from build123d import *

# Parameters (mm, degrees)
SKETCH11_R                             = 2.5
F_25_SERIES_EXTRUSIONS_25_2550_1_DEPTH = 170


with BuildPart() as part:
    # Sketch11 → 25 series extrusions 25-2550(1) (new body)
    with BuildSketch(Plane(origin=(0, 0, 0), x_dir=(-1, 0, 0), z_dir=(0, 1, 0))):
        with BuildLine():
            Line((8.185, 12.5), (-8.185, 12.5))
            ThreePointArc((-8.185, 12.5), (-9.25, 11.435), (-8.185, 10.37))
            Line((-8.185, 10.37), (-6.227198013, 10.37))
            ThreePointArc((-6.227198013, 10.37), (-5.236616214, 9.708114403), (-5.469039527, 8.539643501))
            Line((-5.469039527, 8.539643501), (-8.697639148, 5.311043881))
            ThreePointArc((-8.697639148, 5.311043881), (-9.72768328, 4.622790395), (-10.942703178, 4.381107911))
            Line((-10.942703178, 4.381107911), (-14.057296822, 4.381107911))
            ThreePointArc((-14.057296822, 4.381107911), (-15.27231672, 4.622790395), (-16.302360852, 5.311043881))
            Line((-16.302360852, 5.311043881), (-19.530960473, 8.539643501))
            ThreePointArc((-19.530960473, 8.539643501), (-19.763383786, 9.708114403), (-18.772801987, 10.37))
            Line((-18.772801987, 10.37), (-16.815, 10.37))
            ThreePointArc((-16.815, 10.37), (-15.75, 11.435), (-16.815, 12.5))
            Line((-16.815, 12.5), (-23, 12.5))
            ThreePointArc((-23, 12.5), (-24.414213562, 11.914213562), (-25, 10.5))
            Line((-25, 10.5), (-25, 4.315))
            ThreePointArc((-25, 4.315), (-23.935, 3.25), (-22.87, 4.315))
            Line((-22.87, 4.315), (-22.87, 6.272801987))
            ThreePointArc((-22.87, 6.272801987), (-22.208114403, 7.263383786), (-21.039643501, 7.030960473))
            Line((-21.039643501, 7.030960473), (-17.811043881, 3.802360852))
            ThreePointArc((-17.811043881, 3.802360852), (-17.122790395, 2.77231672), (-16.881107911, 1.557296822))
            Line((-16.881107911, 1.557296822), (-16.881107911, -1.557296822))
            ThreePointArc((-16.881107911, -1.557296822), (-17.122790395, -2.77231672), (-17.811043881, -3.802360852))
            Line((-17.811043881, -3.802360852), (-21.039643501, -7.030960473))
            ThreePointArc((-21.039643501, -7.030960473), (-22.208114403, -7.263383786), (-22.87, -6.272801987))
            Line((-22.87, -6.272801987), (-22.87, -4.315))
            ThreePointArc((-22.87, -4.315), (-23.935, -3.25), (-25, -4.315))
            Line((-25, -4.315), (-25, -10.5))
            ThreePointArc((-25, -10.5), (-24.414213562, -11.914213562), (-23, -12.5))
            Line((-23, -12.5), (-16.815, -12.5))
            ThreePointArc((-16.815, -12.5), (-15.75, -11.435), (-16.815, -10.37))
            Line((-16.815, -10.37), (-18.772801987, -10.37))
            ThreePointArc((-18.772801987, -10.37), (-19.763383786, -9.708114403), (-19.530960473, -8.539643501))
            Line((-19.530960473, -8.539643501), (-16.302360852, -5.311043881))
            ThreePointArc((-16.302360852, -5.311043881), (-15.27231672, -4.622790395), (-14.057296822, -4.381107911))
            Line((-14.057296822, -4.381107911), (-10.942703178, -4.381107911))
            ThreePointArc((-10.942703178, -4.381107911), (-9.72768328, -4.622790395), (-8.697639148, -5.311043881))
            Line((-8.697639148, -5.311043881), (-5.469039527, -8.539643501))
            ThreePointArc((-5.469039527, -8.539643501), (-5.236616214, -9.708114403), (-6.227198013, -10.37))
            Line((-6.227198013, -10.37), (-8.185, -10.37))
            ThreePointArc((-8.185, -10.37), (-9.25, -11.435), (-8.185, -12.5))
            Line((-8.185, -12.5), (8.185, -12.5))
            ThreePointArc((8.185, -12.5), (9.25, -11.435), (8.185, -10.37))
            Line((8.185, -10.37), (6.227198013, -10.37))
            ThreePointArc((6.227198013, -10.37), (5.236616214, -9.708114403), (5.469039527, -8.539643501))
            Line((5.469039527, -8.539643501), (8.697639148, -5.311043881))
            ThreePointArc((8.697639148, -5.311043881), (9.72768328, -4.622790395), (10.942703178, -4.381107911))
            Line((10.942703178, -4.381107911), (14.057296822, -4.381107911))
            ThreePointArc((14.057296822, -4.381107911), (15.27231672, -4.622790395), (16.302360852, -5.311043881))
            Line((16.302360852, -5.311043881), (19.530960473, -8.539643501))
            ThreePointArc((19.530960473, -8.539643501), (19.763383786, -9.708114403), (18.772801987, -10.37))
            Line((18.772801987, -10.37), (16.815, -10.37))
            ThreePointArc((16.815, -10.37), (15.75, -11.435), (16.815, -12.5))
            Line((16.815, -12.5), (23, -12.5))
            ThreePointArc((23, -12.5), (24.414213562, -11.914213562), (25, -10.5))
            Line((25, -10.5), (25, -4.315))
            ThreePointArc((25, -4.315), (23.935, -3.25), (22.87, -4.315))
            Line((22.87, -4.315), (22.87, -6.272801987))
            ThreePointArc((22.87, -6.272801987), (22.208114403, -7.263383786), (21.039643501, -7.030960473))
            Line((21.039643501, -7.030960473), (17.811043881, -3.802360852))
            ThreePointArc((17.811043881, -3.802360852), (17.122790395, -2.77231672), (16.881107911, -1.557296822))
            Line((16.881107911, -1.557296822), (16.881107911, 1.557296822))
            ThreePointArc((16.881107911, 1.557296822), (17.122790395, 2.77231672), (17.811043881, 3.802360852))
            Line((17.811043881, 3.802360852), (21.039643501, 7.030960473))
            ThreePointArc((21.039643501, 7.030960473), (22.208114403, 7.263383786), (22.87, 6.272801987))
            Line((22.87, 6.272801987), (22.87, 4.315))
            ThreePointArc((22.87, 4.315), (23.935, 3.25), (25, 4.315))
            Line((25, 4.315), (25, 10.5))
            ThreePointArc((25, 10.5), (24.414213562, 11.914213562), (23, 12.5))
            Line((23, 12.5), (16.815, 12.5))
            ThreePointArc((16.815, 12.5), (15.75, 11.435), (16.815, 10.37))
            Line((16.815, 10.37), (18.772801987, 10.37))
            ThreePointArc((18.772801987, 10.37), (19.763383786, 9.708114403), (19.530960473, 8.539643501))
            Line((19.530960473, 8.539643501), (16.302360852, 5.311043881))
            ThreePointArc((16.302360852, 5.311043881), (15.27231672, 4.622790395), (14.057296822, 4.381107911))
            Line((14.057296822, 4.381107911), (10.942703178, 4.381107911))
            ThreePointArc((10.942703178, 4.381107911), (9.72768328, 4.622790395), (8.697639148, 5.311043881))
            Line((8.697639148, 5.311043881), (5.469039527, 8.539643501))
            ThreePointArc((5.469039527, 8.539643501), (5.236616214, 9.708114403), (6.227198013, 10.37))
            Line((6.227198013, 10.37), (8.185, 10.37))
            ThreePointArc((8.185, 10.37), (9.25, 11.435), (8.185, 12.5))
        make_face()
        with Locations((-12.5, 0)):
            Circle(SKETCH11_R, mode=Mode.SUBTRACT)
        with Locations((12.5, 0)):
            Circle(SKETCH11_R, mode=Mode.SUBTRACT)
        with BuildLine():
            Line((-1.678781255, 10.37), (1.678781255, 10.37))
            ThreePointArc((1.678781255, 10.37), (2.198638297, 10.16512894), (2.438958165, 9.660678886))
            ThreePointArc((2.438958165, 9.660678886), (2.716823224, 8.564426963), (3.361297928, 7.635110212))
            Line((3.361297928, 7.635110212), (7.191171941, 3.805236199))
            ThreePointArc((7.191171941, 3.805236199), (7.879425427, 2.775192067), (8.121107911, 1.560172169))
            Line((8.121107911, 1.560172169), (8.121107911, -1.560172169))
            ThreePointArc((8.121107911, -1.560172169), (7.879425427, -2.775192067), (7.191171941, -3.805236199))
            Line((7.191171941, -3.805236199), (3.361297928, -7.635110212))
            ThreePointArc((3.361297928, -7.635110212), (2.716823224, -8.564426963), (2.438958165, -9.660678886))
            ThreePointArc((2.438958165, -9.660678886), (2.198638297, -10.16512894), (1.678781255, -10.37))
            Line((1.678781255, -10.37), (-1.678781255, -10.37))
            ThreePointArc((-1.678781255, -10.37), (-2.198638297, -10.16512894), (-2.438958165, -9.660678886))
            ThreePointArc((-2.438958165, -9.660678886), (-2.716823224, -8.564426963), (-3.361297928, -7.635110212))
            Line((-3.361297928, -7.635110212), (-7.191171941, -3.805236199))
            ThreePointArc((-7.191171941, -3.805236199), (-7.879425427, -2.775192067), (-8.121107911, -1.560172169))
            Line((-8.121107911, -1.560172169), (-8.121107911, 1.560172169))
            ThreePointArc((-8.121107911, 1.560172169), (-7.879425427, 2.775192067), (-7.191171941, 3.805236199))
            Line((-7.191171941, 3.805236199), (-3.361297928, 7.635110212))
            ThreePointArc((-3.361297928, 7.635110212), (-2.716823224, 8.564426963), (-2.438958165, 9.660678886))
            ThreePointArc((-2.438958165, 9.660678886), (-2.198638297, 10.16512894), (-1.678781255, 10.37))
        make_face(mode=Mode.SUBTRACT)
    extrude(amount=F_25_SERIES_EXTRUSIONS_25_2550_1_DEPTH)


solid = part.part
Here's how the part is built. I have some questions about the finished solid (model axes, mm). A direction names the side the tool comes from. Give positions to 0.01 mm unless a question says otherwise; leave off trailing zeros. Write each loop counter-clockwise with the first axis right and the second up, starting at its lowest first coordinate (ties: lowest second). Pieces come first, ordered by that corner, then holes. Notation, with made-up numbers: (33, 19) -> (91, 19) arc R9 ccw to (91, 27) -> close; hole circle Ø6 at (67, 41). An arc over 180 degrees is marked (long way). Use one line per item in the form item = value. Start each with the question number.
1. Will these pins go through, and if not, where does the flat tip stop? pin 1 Ø3.5 at (x, y) = (13, 52.5) entering from -Z; pin 2 Ø3.5 at (x, y) = (12, 49) entering from +Z; pin 3 Ø2.5 at (x, y) = (-12.5, 50.5) entering from +Z; pin 4 Ø3 at (x, z) = (-2, -4.5) entering from +Y.
2. Imagine slicing it at B-B on x = 12.5. List the corners of the cut face in (y, z) for me.
3. On a 3-axis mill with a long thin cutter (end or side, diameter ignored), from which of +Z, -Z, +X, -X, +Y, -Y can I reach the whole of each face in a straight line? I mean faces 1 (the face through (-12, 84, -4.381)), 2 (the face through (-7.06, 83.81, -6.95)), 3 (the face through (-16.881, 84, 0)), 4 (the face through (-13, 84, 4.381)). Say none if no direction works.
4. Imagine slicing it at A-A on z = 0. List the corners of the cut face in (x, y) for me, plus the area to 3 significant figures.
5. Thinking about a two-plate mould opening in X: for faces 5 (the face through (19.45, 83.81, 5.44)), 6 (the face through (-20, 84, 12.5)), 7 (the face through (25, 84, 7)), which applies, +X half, -X half, draft (parallel to the pull), parting line (faces both ways), or undercut?
6. If I drill on L1, parallel to X at y = 58.5, z = -0.75; L2, parallel to X at y = 9.5, z = 9; L3, parallel to Z at x = -12.5, y = 52, over which ranges is the centre line in solid material (lowest first)?
7. Imagine slicing it at C-C on y = 79.5. State how many separate pieces and enclosed holes the cut face has, plus the area to 3 significant figures.
Entries:
q1.pin_1 = -4.46
q1.pin_2 = 4.46
q1.pin_3 = 4.38
q1.pin_4 = through
q2.outline = (0, -4.38) -> (170, -4.38) -> (170, -2.5) -> (0, -2.5) -> close; (0, 2.5) -> (170, 2.5) -> (170, 4.38) -> (0, 4.38) -> close
q3.face_1 = -Z, +Y, -Y
q3.face_2 = +Y, -Y
q3.face_3 = -X, +Y, -Y
q3.face_4 = +Z, +Y, -Y
q4.outline = (-16.88, 0) -> (-15, 0) -> (-15, 170) -> (-16.88, 170) -> close; (-10, 0) -> (-8.12, 0) -> (-8.12, 170) -> (-10, 170) -> close; (8.12, 0) -> (10, 0) -> (10, 170) -> (8.12, 170) -> close; (15, 0) -> (16.88, 0) -> (16.88, 170) -> (15, 170) -> close
q4.area = 1,280 mm²
q5.face_5 = undercut
q5.face_6 = draft
q5.face_7 = +X half
q6.L1 = -16.88 to -14.88, -10.12 to -8.12, 8.12 to 10.12, 14.88 to 16.88
q6.L2 = -25 to -19.8, -5.2 to -2.56, 2.56 to 5.2, 19.8 to 25
q6.L3 = -4.38 to -2.5, 2.5 to 4.38
q7.separate_pieces = 1
q7.enclosed_holes = 3
q7.area = 486 mm²
